from build123d import *

# Parameters (mm, degrees)
F1_DEPTH = 2
F2_DEPTH = 12


with BuildPart() as f1:
    # F0 (on Top) → F1 (new body)
    with BuildSketch(Plane.XY):
        with BuildLine():
            ThreePointArc((-68, -25), (-65.071068, -32.071068), (-58, -35))
            Line((-58, -35), (58, -35))
            ThreePointArc((58, -35), (65.071068, -32.071068), (68, -25))
            Line((68, -25), (68, 25))
            ThreePointArc((68, 25), (65.071068, 32.071068), (58, 35))
            Line((58, 35), (-58, 35))
            ThreePointArc((-58, 35), (-65.071068, 32.071068), (-68, 25))
            Line((-68, 25), (-68, -25))
        make_face()
    extrude(amount=F1_DEPTH)

    # F0 (on Top) → F2 (join)
    with BuildSketch(Plane.XY):
        with BuildLine():
            Line((58, 39), (-58, 39))
            ThreePointArc((-58, 39), (-67.899495, 34.899495), (-72, 25))
            Line((-72, 25), (-72, -25))
            ThreePointArc((-72, -25), (-67.899495, -34.899495), (-58, -39))
            Line((-58, -39), (58, -39))
            ThreePointArc((58, -39), (67.899495, -34.899495), (72, -25))
            Line((72, -25), (72, 25))
            ThreePointArc((72, 25), (67.899495, 34.899495), (58, 39))
        make_face()
        with BuildLine():
            Line((58, -35), (-58, -35))
            ThreePointArc((-58, -35), (-65.071068, -32.071068), (-68, -25))
            Line((-68, -25), (-68, 25))
            ThreePointArc((-68, 25), (-65.071068, 32.071068), (-58, 35))
            Line((-58, 35), (58, 35))
            ThreePointArc((58, 35), (65.071068, 32.071068), (68, 25))
            Line((68, 25), (68, -25))
            ThreePointArc((68, -25), (65.071068, -32.071068), (58, -35))
        make_face(mode=Mode.SUBTRACT)
    extrude(amount=F2_DEPTH)


solid = f1.part
Geometry: final body of the model. Coordinates: model frame, mm. A direction names the side the tool comes from. Give positions to 0.01 mm unless a question says otherwise; leave off trailing zeros. Loops run counter-clockwise (first coordinate to the right, second up) from the corner with the lowest first, then second, coordinate; pieces in that order, holes last. Notation, with made-up numbers: (82.25, 49.25) - (132.25, 49.25) arc R13 cw to (132.25, 70.25) - close; hole circle Ø5 at (38, -22.75). An arc over 180 degrees is marked (long way). Answer as CSV lines item,"result". Start each with the question number.
1. Section B-B, the plane y = -2. Return loops of the section in (x, z), plus the area to 3 significant figures.
2. Ray query, L1, parallel to Y at x = -55, z = 3; L2, parallel to X at y = 16, z = 10.5; L3, parallel to Z at x = -35.5, y = -34.5. Return the intervals inside material, ascending.
3. Section C-C, the plane x = 6. Return loops of the section in (y, z).
4. Pin query (flat end, axial travel): P1, Ø12, axis at x = 45, y = -4, coming from the +Z side. Return the tip coordinate at first contact, or that it passes through.
5. Reachability of faces 1 (the face through (1, 39, 6)), 2 (the face through (-68, 0, 7)) from +Z, -Z, +X, -X, +Y, -Y: full face, straight path, thin tool, end or side. Return the list, or none.
6. Draft query along Y for faces 3 (the face through (-1, 1, 0)), 4 (the face through (-1, -39, 6)), 5 (the face through (1, -35, 7)), 6 (the face through (68, 0, 7)). Return one class per face: released by +Y, released by -Y, zero draft, split by the parting line, or undercut.
7. Section A-A, the plane z = 9. Return loops of the section in (x, y).
Answers:
1,outline,"(-72, 0) - (72, 0) - (72, 12) - (68, 12) - (68, 2) - (-68, 2) - (-68, 12) - (-72, 12) - close"
1,area,"368 mm2"
2,L1,"y = -39 to -35, 35 to 39"
2,L2,"x = -72 to -68, 68 to 72"
2,L3,"z = 0 to 2"
3,outline,"(-39, 0) - (39, 0) - (39, 12) - (35, 12) - (35, 2) - (-35, 2) - (-35, 12) - (-39, 12) - close"
4,P1,"stops at z = 2"
5,face 1,"+Z, -Z, +X, -X, +Y"
5,face 2,"+Z"
6,face 3,"zero draft"
6,face 4,"released by -Y"
6,face 5,"undercut"
6,face 6,"undercut"
7,outline,"(-72, -25) arc R14 ccw to (-58, -39) - (58, -39) arc R14 ccw to (72, -25) - (72, 25) arc R14 ccw to (58, 39) - (-58, 39) arc R14 ccw to (-72, 25) - close; hole (-68, -25) arc R10 ccw to (-58, -35) - (58, -35) arc R10 ccw to (68, -25) - (68, 25) arc R10 ccw to (58, 35) - (-58, 35) arc R10 ccw to (-68, 25) - close"
